from build123d import *

# Parameters (mm, degrees)
F0_W     = 10
F0_H     = 4
F1_DEPTH = 22.1
F2_W     = 41.5
F2_H     = 43.485662
F3_DEPTH = 31
F4_R     = 2
F5_R     = 2
F6_R     = 2.5
F7_DEPTH = 25


with BuildPart() as f1:
    # F0 (on Right) → F1 (new body, symmetric)
    with BuildSketch(Plane.YZ):
        with BuildLine():
            Line((-11, 30.769719), (-11, 0))
            Line((-11, 0), (11, 0))
            Line((11, 0), (11, 30.769719))
            ThreePointArc((11, 30.769719), (10.463923, 32.063923), (9.169719, 32.6))
            Line((9.169719, 32.6), (4, 32.6))
            ThreePointArc((4, 32.6), (0, 28.6), (-4, 32.6))
            Line((-4, 32.6), (-9.169719, 32.6))
            ThreePointArc((-9.169719, 32.6), (-10.463923, 32.063923), (-11, 30.769719))
        make_face()
        with Locations((0, 8)):
            Rectangle(F0_W, F0_H, mode=Mode.SUBTRACT)
        with Locations((0, 18)):
            Rectangle(F0_W, F0_H, mode=Mode.SUBTRACT)
    extrude(amount=F1_DEPTH, both=True)

    # F2 (on face) → F3 (cut)
    with BuildSketch(Plane.XY.offset(32.6)):
        with Locations((0, -0.558951)):
            Rectangle(F2_W, F2_H)
    extrude(amount=-F3_DEPTH, mode=Mode.SUBTRACT)

    # F4
    f4_edges = [f1.edges().sort_by_distance(p)[0] for p in [
        (-22.1, 0, 0),
    ]]
    fillet(f4_edges, radius=F4_R)

    # F5
    f5_edges = [f1.edges().sort_by_distance(p)[0] for p in [
        (22.1, 0, 0),
        (-20.75, 0, 1.6),
        (20.75, 0, 1.6),
    ]]
    fillet(f5_edges, radius=F5_R)

    # F6 (on face) → F7 (cut)
    with BuildSketch(Plane.XY.offset(1.6)):
        Circle(F6_R)
    extrude(amount=-F7_DEPTH, mode=Mode.SUBTRACT)


solid = f1.part
Can you work these out from the model? Positions are in its coordinate system, mm. A direction names the side the tool comes from. Coordinates: 2 decimals unless noted, no trailing zeros. Write each loop counter-clockwise with the first axis right and the second up, starting at its lowest first coordinate (ties: lowest second). Pieces come first, ordered by that corner, then holes. Notation, with made-up numbers: (20.25, 86.5) - (26.25, 86.5) arc R36 ccw to (26.25, 125.5) - close; hole circle Ø11 at (-1, 82.25). An arc over 180 degrees is marked (long way). Return JSON: item names as keys, results as strings. Group by question number.
Item 1: I'm going to push flat-ended pins straight in: pin 1 Ø2 at (x, y) = (1.5, 7.5) entering from +Z; pin 2 Ø10 at (x, z) = (12.5, 8.5) entering from +Y; pin 3 Ø0.7 at (x, y) = (21.5, 1) entering from +Z; pin 4 Ø1.1 at (x, y) = (-21.5, 0.5) entering from -Z. Where does each tip first touch, or does it pass through?
Item 2: If we section it at B-B (z = 23.5): Write out the boundary of the cut face in (x, y).
Item 3: Please list where these lines run through material, in increasing order: probe 1 along X at (y, z) = (-0.25, 21.5); probe 2 along Y at (x, z) = (0, 1.2); probe 3 along Z at (x, y) = (10, 6.75).
Item 4: Which directions (+Z, -Z, +X, -X, +Y, -Y) give clear straight access to the entire face, cutting with the end or side of a thin tool? Please do faces 4 (the face through (-20.18, 0.15, 2.2)), 5 (the face through (0.1, 11, 0.5)), 6 (the face through (21, 0, 20)).
Item 5: If we section it at C-C (x = 0): Write out the boundary of the cut face in (y, z), then the cut area to 3 significant figures.
Item 6: If we section it at D-D (z = 18): Write out the boundary of the cut face in (x, y), then the cut area to 3 significant figures.
Item 7: If we section it at A-A (y = 0): Count the separate pieces of the cut face and the enclosed holes in it, then the cut area to 3 significant figures.
Item 8: We'd pull the mould along X, two halves only. Please class faces 1 (the face through (0, 3, 1.6)), 2 (the face through (22.1, 0, 21)), 3 (the face through (21, -5, 18)): pulls with the +X half, pulls with the -X half, needs draft (parallel to the pull), parting line crosses it, or undercut.
Return value:
{
 "1": {"pin 1": "stops at z = 1.6", "pin 2": "passes through", "pin 3": "stops at z = 28.83", "pin 4": "stops at z = 0.19"},
 "2": {"outline": "(-22.1, -11) - (-20.75, -11) - (-20.75, 11) - (-22.1, 11) - close; (20.75, -11) - (22.1, -11) - (22.1, 11) - (20.75, 11) - close"},
 "3": {"probe 1": "x = -22.1 to -20.75, 20.75 to 22.1", "probe 2": "y = -11 to -2.5, 2.5 to 11", "probe 3": "z = 0 to 1.6"},
 "4": {"face 4": "+Z, +Y, -Y", "face 5": "+Z, -Z, +X, -X, +Y", "face 6": "+X, -X"},
 "5": {"outline": "(-11, 0) - (-2.5, 0) - (-2.5, 1.6) - (-11, 1.6) - close; (2.5, 0) - (11, 0) - (11, 1.6) - (2.5, 1.6) - close", "area": "27.2 mm^2"},
 "6": {"outline": "(-22.1, -11) - (-20.75, -11) - (-20.75, -5) - (-22.1, -5) - close; (-22.1, 5) - (-20.75, 5) - (-20.75, 11) - (-22.1, 11) - close; (20.75, -11) - (22.1, -11) - (22.1, -5) - (20.75, -5) - close; (20.75, 5) - (22.1, 5) - (22.1, 11) - (20.75, 11) - close", "area": "32.4 mm^2"},
 "7": {"separate pieces": "6", "enclosed holes": "0", "area": "114 mm^2"},
 "8": {"face 1": "undercut", "face 2": "pulls with the +X half", "face 3": "needs draft"}
}
